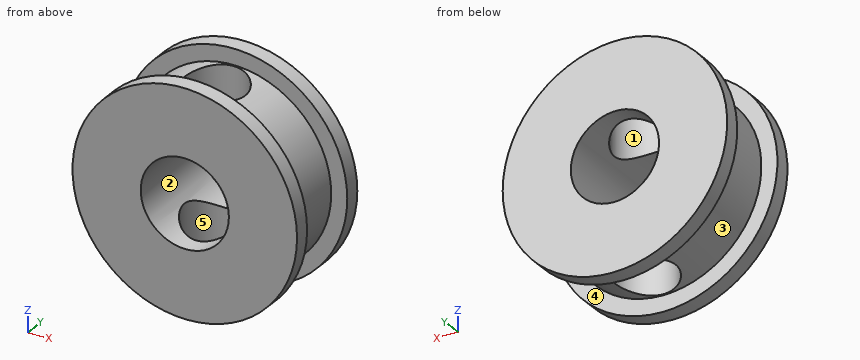
```python
from build123d import *

# Parameters (mm, degrees)
SKETCH_4_R               = 1.9
CUT_EXTRUDE_3_DEPTH      = 8
CUT_EXTRUDE_3_DEPTH_BACK = 8
SKETCH_5_R               = 2.75
CUT_EXTRUDE_4_DEPTH      = 10


with BuildPart() as part:
    # 스케치2 → 회전2 (revolve)
    with BuildSketch(Plane.XY):
        Polygon((0, 3.263948498), (7, 3.263948498), (7, 2.263948498), (6, 2.263948498), (6, -1.736051502), (7, -1.736051502), (7, -2.736051502), (0, -2.736051502), align=None)
    revolve(axis=Axis((0, 3.263948498, 0), (0, -1, 0)))

    # 스케치4 → 컷-돌출3 (cut, two sides)
    with BuildSketch(Plane.XY) as cut_extrude_3_sk:
        with Locations((0, 0.263948498)):
            Circle(SKETCH_4_R)
    extrude(amount=CUT_EXTRUDE_3_DEPTH, mode=Mode.SUBTRACT)
    extrude(cut_extrude_3_sk.sketch, amount=-CUT_EXTRUDE_3_DEPTH_BACK, mode=Mode.SUBTRACT)

    # 스케치5 → 컷-돌출4 (cut)
    with BuildSketch(Plane(origin=(0, 3.263948498, 0), x_dir=(1, 0, 0), z_dir=(0, 1, 0))):
        Circle(SKETCH_5_R)
    extrude(amount=-CUT_EXTRUDE_4_DEPTH, mode=Mode.SUBTRACT)


solid = part.part
```
Verification items for the finished model (mm, model axes). Face numbers are marked on the shaded views. A direction names the side the tool comes from. Coordinates: 2 decimals unless noted, no trailing zeros. Loops run counter-clockwise (first coordinate to the right, second up) from the corner with the lowest first, then second, coordinate; pieces in that order, holes last. Notation, with made-up numbers: (-1.75, 17.25) - (2.25, 17.25) arc R6 ccw to (2.25, 21.25) - close; hole circle Ø11 at (17, 61.5). An arc over 180 degrees is marked (long way). Answer as a JSON object with one key per item and string values.
(1) Access from +Z, -Z, +X, -X, +Y, -Y to the whole of each face (thin tool, end or side, straight path). Record for the marked faces 4 and 5.
Response:
{"face 4": "none", "face 5": "+Z, -Z"}
(2) Cross-section at B-B, the plane x = 0. Record the boundary of the cut face in (y, z), then the cut area to 3 significant figures.
Response:
{"outline": "(-2.74, -7) - (-1.74, -7) - (-1.74, -6) - (-1.64, -6) - (-1.64, -2.75) - (-2.74, -2.75) - close; (-2.74, 2.75) - (-1.64, 2.75) - (-1.64, 6) - (-1.74, 6) - (-1.74, 7) - (-2.74, 7) - close; (2.16, -6) - (2.26, -6) - (2.26, -7) - (3.26, -7) - (3.26, -2.75) - (2.16, -2.75) - close; (2.16, 2.75) - (3.26, 2.75) - (3.26, 7) - (2.26, 7) - (2.26, 6) - (2.16, 6) - close", "area": "18.3 mm²"}
(3) Cross-section at D-D, the plane y = 3. Record the boundary of the cut face in (x, z).
Response:
{"outline": "circle Ø14 at (0, 0); hole circle Ø5.5 at (0, 0)"}
(4) Mould release check, pull along Z, two halves, no side actions. Record for the marked faces 1, 2 and 3: pulls with the +Z half, pulls with the -Z half, needs draft (parallel to the pull), parting line crosses it, or undercut.
Response:
{"face 1": "needs draft", "face 2": "undercut", "face 3": "parting line crosses it"}
(5) Cross-section at C-C, the plane y = 1.5. Record the boundary of the cut face in (x, z).
Response:
{"outline": "(-1.44, -5.82) - (-1.44, -2.34) arc R2.75 cw to (-1.44, 2.34) - (-1.44, 5.82) arc R6 ccw to start; (1.44, -5.82) arc R6 ccw to (1.44, 5.82) - (1.44, 2.34) arc R2.75 cw to (1.44, -2.34) - close"}
(6) Go/stop test with flat-tipped pins: pin 1 Ø6.5 at (x, z) = (0, 0) entering from +Y; pin 2 Ø3.5 at (x, y) = (0, 0.26) entering from -Z. Record where each tip stops, or that it passes through.
Response:
{"pin 1": "stops at y = 3.26", "pin 2": "passes through"}
(7) Scan lines: line 1 along Y through (x, z) = (-5.5, 4); line 2 along Y through (x, z) = (0, -4.1); line 3 along X through (y, z) = (-0.5, 1). Record each from-to range of solid material in increasing order.
Response:
{"line 1": "y = -2.74 to -1.74, 2.26 to 3.26", "line 2": "y = -2.74 to -1.64, 2.16 to 3.26", "line 3": "x = -5.92 to -2.56, 2.56 to 5.92"}
(8) Cross-section at A-A, the plane z = 0. Record the boundary of the cut face in (x, y), then the cut area to 3 significant figures.
Response:
{"outline": "(-7, -2.74) - (-2.75, -2.74) - (-2.75, 3.26) - (-7, 3.26) - (-7, 2.26) - (-6, 2.26) - (-6, -1.74) - (-7, -1.74) - close; (2.75, -2.74) - (7, -2.74) - (7, -1.74) - (6, -1.74) - (6, 2.26) - (7, 2.26) - (7, 3.26) - (2.75, 3.26) - close", "area": "43.0 mm²"}
